Geometry check sheet. Reference: the model listing, model coordinates, mm. Give positions to 0.01 mm unless a question says otherwise; leave off trailing zeros. Write each loop counter-clockwise with the first axis right and the second up, starting at its lowest first coordinate (ties: lowest second). Pieces come first, ordered by that corner, then holes. Notation, with made-up numbers: (12, -11.5) -> (57, -11.5) arc R33 ccw to (57, 24.5) -> close; hole circle Ø9 at (56.5, 2.5). An arc over 180 degrees is marked (long way). Write item = value, one per line. Start each with the question number.
1. Cross-section at A-A, the plane x = 0. Record the cut outline in (y, z) (3 decimals).
2. Cross-section at B-B, the plane y = 0. Record the cut outline in (x, z) (3 decimals), plus the area to 3 significant figures.
3. Depth check by flat-ended pin: P1, Ø4, axis at y = 7, z = 8.5, coming from the +X side; P2, Ø1.5, axis at y = 5, z = 4.5, coming from the +X side; P3, Ø1, axis at y = -6.5, z = 12, coming from the +X side. Enter the tip coordinate at first touch or a pass-through.
4. Cross-section at C-C, the plane x = 8. Record the cut outline in (y, z), plus the area to 3 significant figures.
5. Thickness scan on line 1 along Y through (x, z) = (4.75, 11.75); line 2 along Y through (x, z) = (2.5, 13.75); line 3 along X through (y, z) = (-22, 5.5). Record the ranges inside material, lowest first.
6. Mould release check, pull along Y, two halves, no side actions. Record for faces 1 (the flat face through (0, -11, 0)), 2 (the cylindrical face through (0.399, 12.694, 9.392)): pulls with the +Y half, pulls with the -Y half, needs draft (parallel to the pull), parting line crosses it, or undercut.
7. Cross-section at D-D, the plane y = -26. Record the cut outline in (x, z) (3 decimals), plus the area to 3 significant figures.
```python
from build123d import *

# Parameters (mm, degrees)
F0_R     = 9.525
F1_DEPTH = 19.05
F2_R     = 5.08


with BuildPart() as f1:
    # F0 (on Top) → F1 (new body)
    with BuildSketch(Plane.XY):
        with BuildLine():
            ThreePointArc((-6.1483610621, -11.1125), (0, -34.925), (6.1483610621, -11.1125))
            ThreePointArc((6.1483610621, -11.1125), (0, 12.7), (-6.1483610621, -11.1125))
        make_face()
        with Locations((0, -22.225)):
            Circle(F0_R, mode=Mode.SUBTRACT)
        Circle(F0_R, mode=Mode.SUBTRACT)
    extrude(amount=F1_DEPTH)

    # F2
    f2_edges = [f1.edges().sort_by_distance(p)[0] for p in [
        (6.148361, -11.1125, 9.525),
        (-6.148361, -11.1125, 9.525),
    ]]
    fillet(f2_edges, radius=F2_R)


solid = f1.part
```
Answers:
q1.outline = (-34.925, 0) -> (-31.75, 0) -> (-31.75, 19.05) -> (-34.925, 19.05) -> close; (-12.7, 0) -> (-9.525, 0) -> (-9.525, 19.05) -> (-12.7, 19.05) -> close; (9.525, 0) -> (12.7, 0) -> (12.7, 19.05) -> (9.525, 19.05) -> close
q2.outline = (-12.7, 0) -> (-9.525, 0) -> (-9.525, 19.05) -> (-12.7, 19.05) -> close; (9.525, 0) -> (12.7, 0) -> (12.7, 19.05) -> (9.525, 19.05) -> close
q2.area = 121 mm^2
q3.P1 = 11.67
q3.P2 = 11.97
q3.P3 = 11.19
q4.outline = (-32.09, 0) -> (-27.39, 0) -> (-27.39, 19.05) -> (-32.09, 19.05) -> close; (-17.06, 0) -> (-5.17, 0) -> (-5.17, 19.05) -> (-17.06, 19.05) -> close; (5.17, 0) -> (9.86, 0) -> (9.86, 19.05) -> (5.17, 19.05) -> close
q4.area = 405 mm^2
q5.line_1 = -34 to -30.48, -13.97 to -8.26, 8.26 to 11.78
q5.line_2 = -34.68 to -31.42, -13.03 to -9.19, 9.19 to 12.45
q5.line_3 = -12.7 to -9.52, 9.52 to 12.7
q6.face_1 = needs draft
q6.face_2 = undercut
q7.outline = (-12.126, 0) -> (-8.745, 0) -> (-8.745, 19.05) -> (-12.126, 19.05) -> close; (8.745, 0) -> (12.126, 0) -> (12.126, 19.05) -> (8.745, 19.05) -> close
q7.area = 129 mm^2
